Autodesk Inventor part; units mm, degrees
ref_plane "YZ Plane" through (0, 0, 0) normal (1, 0, 0) x (0, 1, 0)
ref_plane "XZ Plane" through (0, 0, 0) normal (0, 1, 0) x (-1, 0, 0)
ref_plane "XY Plane" through (0, 0, 0) normal (0, 0, 1) x (1, 0, 0)
sketch "Sketch1" plane through (0, 0, 0) normal (0, 1, 0) x (-1, 0, 0)
  line L0 (0, 0) -> (7.62, 0)
  line L1 (7.62, 0) -> (7.62, -16.51)
  line L2 (7.62, -16.51) -> (0, -16.51)
  line L3 (0, -16.51) -> (0, 0)
  line L4 (0, 0) -> (0, -5.715)
  line L5 (0, -5.715) -> (-7.112, -5.715)
  line L6 (-7.112, -5.715) -> (-7.112, -10.795)
  line L7 (-7.112, -10.795) -> (0, -10.795)
  line L8 (-7.112, -5.715) -> (-4.572, -5.715)
  line L9 (-4.572, -5.715) -> (-4.572, -3.175)
  line L10 (-4.572, -3.175) -> (-7.112, -5.715)
  line L11 (-7.112, -10.795) -> (-4.572, -10.795)
  line L12 (-4.572, -10.795) -> (-4.572, -13.335)
  line L13 (-4.572, -13.335) -> (-7.112, -10.795)
  dimension "d0" = 7.62
  dimension "d1" = 16.51
  dimension "d2" = 5.715
  dimension "d3" = 7.112
  dimension "d4" = 5.08
  dimension "d5" = 2.54
  dimension "d6" = 2.54
  dimension "d7" = 2.54
extrude "Extrusion1" add sketch "Sketch1" along normal blind 25.4
sketch "Sketch2" plane through (0, 25.4, 0) normal (0, 1, 0) x (1, 0, 0)
  line L0 (-7.62, 0) -> (0, 0)
  line L1 (-3.81, 0) -> (-3.81, 4.064)
  line L2 (0, 16.51) -> (-7.62, 16.51)
  line L3 (-3.81, 16.51) -> (-3.81, 12.446)
  circle A0 centre (-3.81, 4.064) radius 1.397
  circle A1 centre (-3.81, 12.446) radius 1.397
  dimension "d10" = 4.064
  dimension "d11" = 4.064
  dimension "d12" = 2.794
  dimension "d13" = 2.794
extrude "Extrusion2" add sketch "Sketch2" along normal blind 2.54
sketch "Sketch3" plane through (0, 25.4, 0) normal (0, 1, 0) x (1, 0, 0)
  line L0 (-7.62, 0) -> (0, 0)
  line L1 (-3.81, 0) -> (-3.81, 8.255)
  dimension "d16" = 8.255
hole "Hole1" at (-3.81, 25.4, -8.255) direction (0, -1, 0) diameter 2.794 depth 11.43 tip angle 118
sketch "Sketch8" plane through (-7.62, 0, 0) normal (0, 0, 1) x (1, 0, 0)
  line L0 (0, 0) -> (6.35, 0)
  line L1 (6.35, 0) -> (6.35, 10.16)
  line L2 (6.35, 10.16) -> (0, 10.16)
  line L3 (0, 10.16) -> (0, 0)
  point P0 (7.62, 0)
  dimension "d43" = 6.35
  dimension "d44" = 10.16
extrude "Extrusion6" add sketch "Sketch8" along normal blind 30.48
sketch "Sketch9" plane through (-1.27, 0, 0) normal (1, 0, 0) x (0, 0, -1)
  line L0 (16.51, 0) -> (-30.48, 0)
  line L1 (0, 10.16) -> (-30.48, 10.16)
  line L2 (-30.48, 0) -> (-20.32, 0)
  line L3 (-20.32, 0) -> (-20.32, 10.16)
  line L4 (-20.32, 10.16) -> (-30.48, 10.16)
  line L5 (-30.48, 10.16) -> (-30.48, 0)
  point P0 (0, 0)
  point P1 (46.99, 0)
  dimension "d47" = 10.16
extrude "Extrusion7" add sketch "Sketch9" along normal blind 44.45
sketch "Sketch10" plane through (43.18, 0, 0) normal (1, 0, 0) x (0, 0, -1)
  line L0 (-20.32, 10.16) -> (-20.32, 0)
  line L1 (-20.32, 5.08) -> (-25.4, 5.08)
  circle A0 centre (-25.4, 5.08) radius 2.54
  point P0 (0, 0)
  dimension "d50" = 5.08
  dimension "d51" = 5.08
extrude "Extrusion8" add sketch "Sketch10" along normal blind 7.62
sketch "Sketch11" plane through (50.8, 5.08, 25.4) normal (1, 0, 0) x (0, 0, -1)
  circle A0 centre (0, 0) radius 1.397
  point P0 (25.4, -5.08)
  dimension "d54" = 2.794
hole "Hole3" at (50.8, 5.08, 25.4) direction (-1, 0, 0) diameter 2.794 depth 16.002 tip angle 118
properties part number "Grab Rail v2"
For this review, take the finished solid that the model builds, in its own axes (mm). A direction names the side the tool comes from. Coordinates: 2 decimals unless noted, no trailing zeros. Loops run counter-clockwise (first coordinate to the right, second up) from the corner with the lowest first, then second, coordinate; pieces in that order, holes last. Notation, with made-up numbers: (21, 34.25) -> (42, 34.25) arc R20 ccw to (42, 39.25) -> close; hole circle Ø8 at (60.5, 47.5). An arc over 180 degrees is marked (long way). Return JSON: item names as keys, results as strings. Group by question number.
(1) Consider section C-C, the plane x = 38. Give the boundary of the cut face in (y, z), plus the area to 3 significant figures.
(2) Consider section D-D, the plane z = 6. Give the boundary of the cut face in (x, y), plus the area to 3 significant figures.
(3) To check wall thickness, follow L1, parallel to Z at x = -3.81, y = 23.25; L2, parallel to Z at x = 38.75, y = 5.08; L3, parallel to Y at x = 44.75, z = 25.4. State the ranges of each line that lie inside material, in increasing order.
(4) For pin 1 Ø11 at (x, y) = (23.5, 5) entering from -Z; pin 2 Ø1.4 at (x, y) = (3, 13) entering from -Z (3 decimals); pin 3 Ø6.5 at (y, z) = (9, -13) entering from +X; pin 4 Ø4 at (y, z) = (19, 3) entering from +X, all flat-tipped, find the tip position at first contact; note any pin that passes through.
(5) Consider section B-B, the plane y = 9. Give the boundary of the cut face in (x, z) (3 decimals), plus the area to 3 significant figures.
(6) Mouldability with a two-part tool opening along Y and no side actions: class faces 5 (the conical face through (-3.903, 13.276, -8.031)), 6 (the cylindrical face through (42.687, 4.136, 26.43)), 7 (the flat face through (5.824, 12.522, -12.083)) as pulls with the +Y half, pulls with the -Y half, needs draft (parallel to the pull), parting line crosses it, or undercut.
(7) Consider section A-A, the plane y = 21.75. Give the boundary of the cut face in (x, z) (3 decimals), plus the area to 3 significant figures.
(8) Tool access review of faces 1 (the flat face through (-1.27, 5, 10)), 2 (the cylindrical face through (-2.57, 19.6, -7.61)), 3 (the flat face through (2, 13, -10.795)), 4 (the flat face through (-3, 15, 0)): name each direction out of +Z, -Z, +X, -X, +Y, -Y from which nothing blocks a thin tool from reaching the whole face with its end or side.
Results below:
{
 "1": {"outline": "(0, 20.32) -> (10.16, 20.32) -> (10.16, 30.48) -> (0, 30.48) -> close; hole circle Ø2.79 at (5.08, 25.4)", "area": "97.1 mm2"},
 "2": {"outline": "(-7.62, 0) -> (-1.27, 0) -> (-1.27, 10.16) -> (-7.62, 10.16) -> close", "area": "64.5 mm2"},
 "3": {"L1": "z = -16.51 to -9.65, -6.86 to 0", "L2": "z = 20.32 to 24, 26.8 to 30.48", "L3": "y = 2.54 to 3.68, 6.48 to 7.62"},
 "4": {"pin 1": "stops at z = 20.32", "pin 2": "stops at z = -10.795", "pin 3": "stops at x = 7.11", "pin 4": "passes through"},
 "5": {"outline": "(-7.62, -16.51) -> (0, -16.51) -> (0, -10.795) -> (4.572, -10.795) -> (4.572, -13.335) -> (7.112, -10.795) -> (7.112, -5.715) -> (4.572, -3.175) -> (4.572, -5.715) -> (0, -5.715) -> (0, 0) -> (-1.27, 0) -> (-1.27, 20.32) -> (43.18, 20.32) -> (43.18, 30.48) -> (-7.62, 30.48) -> close", "area": "814 mm2"},
 "6": {"face 5": "pulls with the +Y half", "face 6": "undercut", "face 7": "needs draft"},
 "7": {"outline": "(-7.62, -16.51) -> (0, -16.51) -> (0, -10.795) -> (4.572, -10.795) -> (4.572, -13.335) -> (7.112, -10.795) -> (7.112, -5.715) -> (4.572, -3.175) -> (4.572, -5.715) -> (0, -5.715) -> (0, 0) -> (-7.62, 0) -> close; hole circle Ø2.794 at (-3.81, -8.255)", "area": "162 mm2"},
 "8": {"face 1": "+X, +Y, -Y", "face 2": "+Y", "face 3": "-Z, +Y, -Y", "face 4": "+X, +Y"}
}
